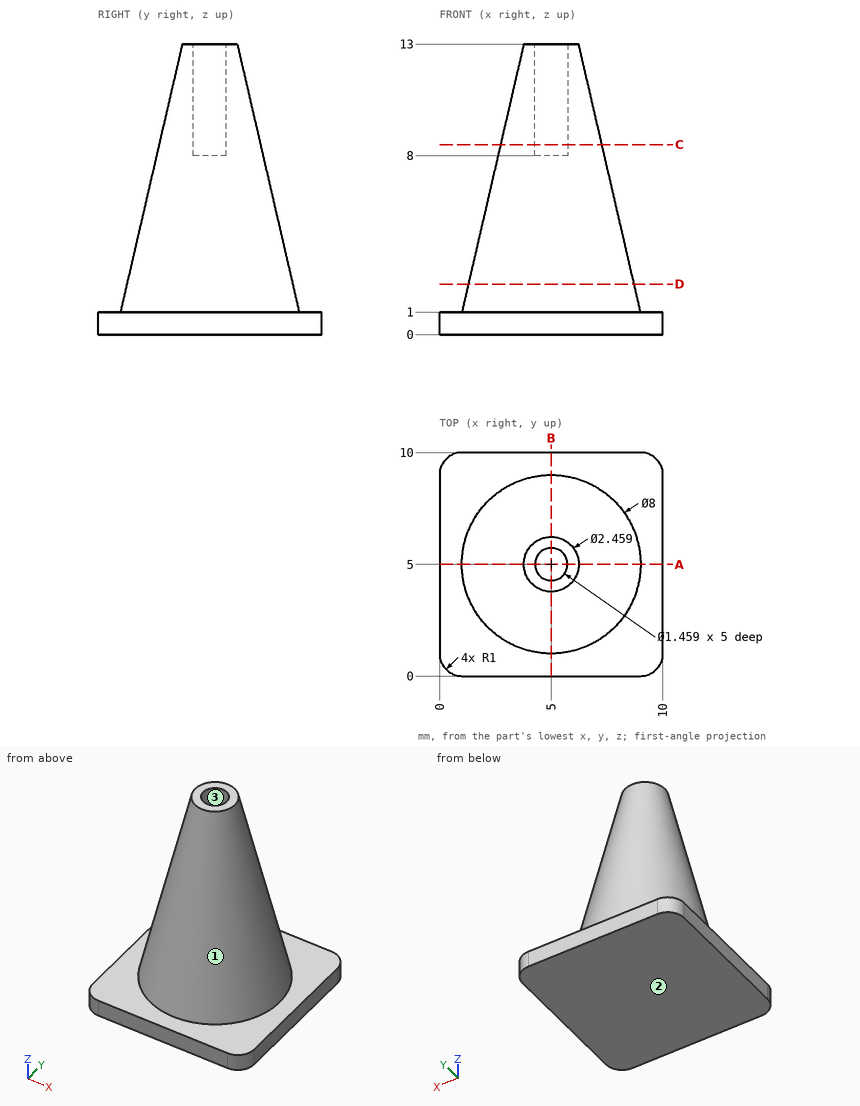
Job drawing, mm, ordinate dimensions from the low corner. One solid piece. Coordinates: 2 decimals unless noted, no trailing zeros. Order: outer loops, then holes, each group sorted by start corner. A loop starts at its lowest first (then second) coordinate and runs counter-clockwise, first axis right, second up. Notation, with made-up numbers: (11.25, -0.75) - (60.25, -0.75) arc R21 cw to (60.25, 33.25) - close; hole circle Ø9 at (50, -18). An arc over 180 degrees is marked (long way). Write each question's results on one line, items separated by ' | '. Start each with the question number.
Item 1: Band-saw the part on A-A on y = 5. Write the cut outline in (x, z).
Item 2: Mould opens along X. For the marked faces 1, 2 and 3 say: released by +X, released by -X, zero draft, split by the parting line, or undercut.
Item 3: Band-saw the part on D-D on z = 2.25. Write the cut outline in (x, y).
Item 4: Flat gauge pins, fed straight in: pin 1 (4 mm diameter, centred on y = 6, z = 10.5, fed in from -X); pin 2 (1 mm diameter, centred on y = 3.5, z = 5.5, fed in from -X). Where does each tip first touch, or does it go through?
Item 5: Band-saw the part on C-C on z = 8.5. Write the cut outline in (x, y), and give its area (3 significant figures).
Item 6: Wall check: probe 1 along Z at (x, y) = (0.75, 9); probe 2 along Y at (x, z) = (5, 11.45); probe 3 along Y at (x, z) = (5, 11.05). Give the ranges that are in metal, low to high. Write a range as [from, to].
Numbers:
1) outline: (0, 0) - (10, 0) - (10, 1) - (9, 1) - (6.23, 13) - (5.73, 13) - (5.73, 8) - (4.27, 8) - (4.27, 13) - (3.77, 13) - (1, 1) - (0, 1) - close
2) face 1: split by the parting line | face 2: zero draft | face 3: undercut
3) outline: circle Ø7.42 at (5, 5)
4) pin 1: x = 2.78 | pin 2: x = 2.18
5) outline: circle Ø4.54 at (5, 5); hole circle Ø1.46 at (5, 5) | area: 14.5 mm^2
6) probe 1: [0, 1] | probe 2: [3.41, 4.27], [5.73, 6.59] | probe 3: [3.32, 4.27], [5.73, 6.68]
